Work out the finished part from the listing and answer in its coordinate system (mm). Face numbers are marked on the shaded views. A direction names the side the tool comes from. Coordinates: 2 decimals unless noted, no trailing zeros. Loops run counter-clockwise (first coordinate to the right, second up) from the corner with the lowest first, then second, coordinate; pieces in that order, holes last. Notation, with made-up numbers: (38.5, -11) - (87.5, -11) arc R19 cw to (87.5, 20) - close; hole circle Ø4 at (35, 22.5). An arc over 180 degrees is marked (long way). Write each question's results on one line, items separated by ' | '. Start each with the question number.
Item 1: A tool of negligible diameter and unlimited length cuts with its end or side. For the marked faces 4, 5, 6, 7 and 8, from which of +Z, -Z, +X, -X, +Y, -Y can it reach the whole face along a straight path? Write none if from no direction.
Item 2: Section B-B, the plane y = -327 is taken. Write down the section's boundary in (x, z), plus the area to 3 significant figures.
Item 3: Each of these flat-tipped pins is pushed along its axis until it touches: pin 1 Ø6 at (x, y) = (-10, -240) entering from +Z; pin 2 Ø3.5 at (x, z) = (-109, -55) entering from -Y; pin 3 Ø1.5 at (y, z) = (-158, -40) entering from -X; pin 4 Ø5 at (x, z) = (-7, -40) entering from -Y. Where does it stop, or does it pass through?
Item 4: For a pull along Y with two mould halves and no side action, classify the marked faces 1, 2 and 3 as +Y half, -Y half, draft (parallel to the pull), parting line (faces both ways), or undercut.
Item 5: Section A-A, the plane z = -15 is taken. Write down the section's boundary in (x, y).
Item 6: Consider probe 1 along X at (y, z) = (-395, -25); probe 2 along X at (y, z) = (6.75, -15); probe 3 along Y at (x, z) = (-20, -33.5). Determine where each line is inside the solid, lowest interval first. Write a range as [from, to].
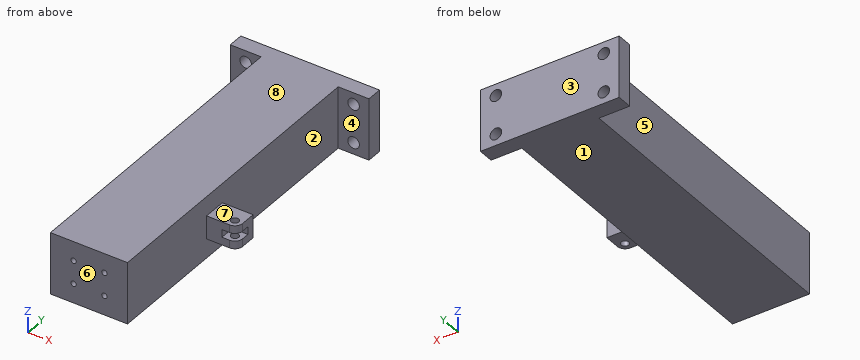
from build123d import *

# Parameters (mm, degrees)
SKETCH1_W           = 180
SKETCH1_H           = 80
BOSS_EXTRUDE1_DEPTH = 20
SKETCH2_R           = 7.5
CUT_EXTRUDE1_DEPTH  = 198.989898732
SKETCH3_W           = 100
SKETCH3_H           = 80
BOSS_EXTRUDE2_DEPTH = 400
SKETCH4_R           = 3.5
CUT_EXTRUDE2_DEPTH  = 10
SKETCH12_W          = 30
SKETCH12_H          = 30
BOSS_EXTRUDE6_DEPTH = 40
SKETCH13_R          = 5
CUT_EXTRUDE7_DEPTH  = 30
SKETCH14_W          = 10
SKETCH14_H          = 20
CUT_EXTRUDE8_DEPTH  = 20
FILLET4_R           = 10


with BuildPart() as part:
    # Sketch1 → Boss-Extrude1 (new body)
    with BuildSketch(Plane(origin=(0, 0, 0), x_dir=(1, 0, 0), z_dir=(0, 1, 0))):
        with Locations((-90, 40)):
            Rectangle(SKETCH1_W, SKETCH1_H)
    extrude(amount=BOSS_EXTRUDE1_DEPTH)

    # Sketch2 → Cut-Extrude1 (cut, through all)
    with BuildSketch(Plane(origin=(0, 20, 0), x_dir=(1, 0, 0), z_dir=(0, 1, 0))):
        with Locations(Location((-160, 65, 0), (0, 0, 270))):
            Circle(SKETCH2_R)
        with Locations(Location((-160, 15, 0), (0, 0, 270))):
            Circle(SKETCH2_R)
        with Locations(Location((-20, 65, 0), (0, 0, 270))):
            Circle(SKETCH2_R)
        with Locations(Location((-20, 15, 0), (0, 0, 270))):
            Circle(SKETCH2_R)
    extrude(amount=-CUT_EXTRUDE1_DEPTH, mode=Mode.SUBTRACT)

    # Sketch3 → Boss-Extrude2 (add)
    with BuildSketch(Plane.XZ):
        with Locations((-90, -40)):
            Rectangle(SKETCH3_W, SKETCH3_H)
    extrude(amount=BOSS_EXTRUDE2_DEPTH)

    # Sketch4 → Cut-Extrude2 (cut)
    with BuildSketch(Plane.XZ.offset(400)):
        with Locations(Location((-110, -25, 0), (0, 0, 270))):
            Circle(SKETCH4_R)
        with Locations(Location((-70, -25, 0), (0, 0, 270))):
            Circle(SKETCH4_R)
        with Locations(Location((-110, -55, 0), (0, 0, 270))):
            Circle(SKETCH4_R)
        with Locations(Location((-70, -55, 0), (0, 0, 270))):
            Circle(SKETCH4_R)
    extrude(amount=-CUT_EXTRUDE2_DEPTH, mode=Mode.SUBTRACT)

    # Sketch12 → Boss-Extrude6 (add)
    with BuildSketch(Plane(origin=(-40, 0, 0), x_dir=(0, 0, -1), z_dir=(1, 0, 0))):
        with Locations((40, -235)):
            Rectangle(SKETCH12_W, SKETCH12_H)
    extrude(amount=BOSS_EXTRUDE6_DEPTH)

    # Sketch13 → Cut-Extrude7 (cut)
    with BuildSketch(Plane.XY.offset(-25)):
        with Locations((-10, -240)):
            Circle(SKETCH13_R)
    extrude(amount=-CUT_EXTRUDE7_DEPTH, mode=Mode.SUBTRACT)

    # Sketch14 → Cut-Extrude8 (cut)
    with BuildSketch(Plane(origin=(0, 0, 0), x_dir=(0, 0, -1), z_dir=(1, 0, 0))):
        with Locations((40, -240)):
            Rectangle(SKETCH14_W, SKETCH14_H)
    extrude(amount=-CUT_EXTRUDE8_DEPTH, mode=Mode.SUBTRACT)

    # Fillet4
    fillet4_edges = [part.edges().sort_by_distance(p)[0] for p in [
        (0, -250, -30),
        (0, -250, -50),
        (-20, -230, -40),
    ]]
    fillet(fillet4_edges, radius=FILLET4_R)


solid = part.part
Answer key:
1) face 4: +Z, -Z, +X | face 5: +Z, -Z, -X, -Y | face 6: +Z, -Z, +X, -X, -Y | face 7: +Z, +X, -Y | face 8: +Z, +X, -X, +Y, -Y
2) outline: (-140, -80) - (-40, -80) - (-40, 0) - (-140, 0) - close | area: 8,000 mm^2
3) pin 1: passes through | pin 2: stops at y = -390 | pin 3: stops at x = -140 | pin 4: stops at y = -230
4) face 1: draft | face 2: undercut | face 3: +Y half
5) outline: (-180, 0) - (-167.5, 0) - (-167.5, 20) - (-180, 20) - close; (-152.5, 0) - (-140, 0) - (-140, -400) - (-40, -400) - (-40, 0) - (-27.5, 0) - (-27.5, 20) - (-152.5, 20) - close; (-12.5, 0) - (0, 0) - (0, 20) - (-12.5, 20) - close
6) probe 1: x = [-140, -113.5], [-106.5, -73.5], [-66.5, -40] | probe 2: x = [-180, -167.5], [-152.5, -27.5], [-12.5, 0] | probe 3: y = [-250, -220], [0, 20]
